from build123d import *

# Parameters (mm, degrees)
SKETCH1_R           = 3.2639
BOSS_EXTRUDE1_DEPTH = 6.35
FILLET2_R           = 6.35
FILLET3_R           = 2.54
FILLET6_R           = 6.35
FILLET7_R           = 6.35


with BuildPart() as part:
    # Sketch1 → Boss-Extrude1 (new, symmetric)
    with BuildSketch(Plane.XY):
        with BuildLine():
            ThreePointArc((1657.362226857, -25.665303386), (1645.082138382, -19.376819434), (1639.161234094, -31.838299916))
            Line((1639.161234094, -31.838299916), (1543.928298612, -110.961407638))
            Line((1543.928298612, -110.961407638), (1542.386268966, -109.105413681))
            Line((1542.386268966, -109.105413681), (1475.716388889, -164.497259751))
            ThreePointArc((1475.716388889, -164.497259751), (1463.735668917, -172.561408735), (1473.270132637, -183.40862734))
            Line((1473.270132637, -183.40862734), (1482.795132637, -183.40862734))
            Line((1482.795132637, -183.40862734), (1536.006430236, -216.269775409))
            Line((1536.006430236, -216.269775409), (1475.438186342, -259.678478553))
            ThreePointArc((1475.438186342, -259.678478553), (1465.455879345, -274.64513078), (1482.83634148, -270.00113812))
            Line((1482.83634148, -270.00113812), (1554.239311773, -218.827286252))
            Line((1554.239311773, -218.827286252), (1553.129588502, -217.278887316))
            Line((1553.129588502, -217.278887316), (1710.323691942, -104.61931964))
            Line((1710.323691942, -104.61931964), (1709.583876428, -103.587053683))
            Line((1709.583876428, -103.587053683), (1795.041714347, -42.340207499))
            ThreePointArc((1795.041714347, -42.340207499), (1809.776954687, -31.712536315), (1791.625246623, -30.944293485))
            Line((1791.625246623, -30.944293485), (1657.362226857, -25.665303386))
        make_face()
        with BuildLine():
            Line((1700.720652168, -102.126820321), (1556.109252329, -109.096723899))
            Line((1556.109252329, -109.096723899), (1643.219206848, -36.72249454))
            ThreePointArc((1643.219206848, -36.72249454), (1647.101886478, -38.035715693), (1651.178708707, -37.612311142))
            Line((1651.178708707, -37.612311142), (1700.720652168, -102.126820321))
        make_face(mode=Mode.SUBTRACT)
        with BuildLine():
            ThreePointArc((1482.659265028, -175.861431519), (1482.859244436, -174.484660756), (1482.858420935, -173.093442291))
            Line((1482.858420935, -173.093442291), (1541.633109373, -124.261218638))
            Line((1541.633109373, -124.261218638), (1541.60005002, -212.260879574))
            Line((1541.60005002, -212.260879574), (1482.659265028, -175.861431519))
        make_face(mode=Mode.SUBTRACT)
        with Locations((1473.270132637, -269.04472734)):
            Circle(SKETCH1_R, mode=Mode.SUBTRACT)
        with Locations((1473.270132637, -173.79472734)):
            Circle(SKETCH1_R, mode=Mode.SUBTRACT)
        Polygon((1547.986271365, -115.845602263), (1688.873329523, -109.05520253), (1547.950879905, -210.053025619), align=None, mode=Mode.SUBTRACT)
        with Locations((1648.169999473, -28.481334088)):
            Circle(SKETCH1_R, mode=Mode.SUBTRACT)
        with BuildLine():
            Line((1705.884798859, -98.425723899), (1656.215061092, -33.744798419))
            ThreePointArc((1656.215061092, -33.744798419), (1656.708059099, -32.900452896), (1657.112748585, -32.010400752))
            Line((1657.112748585, -32.010400752), (1791.19818023, -37.282408394))
            Line((1791.19818023, -37.282408394), (1705.884798859, -98.425723899))
        make_face(mode=Mode.SUBTRACT)
        with Locations((1800.567995736, -34.473360149)):
            Circle(SKETCH1_R, mode=Mode.SUBTRACT)
    extrude(amount=BOSS_EXTRUDE1_DEPTH, both=True)

    # Fillet2
    fillet2_edges = [part.edges().sort_by_distance(p)[0] for p in [
        (1541.60005002, -212.260879574, 0),
        (1547.986271365, -115.845602263, 0),
        (1700.720652168, -102.126820321, 0),
        (1791.625246623, -30.944293485, 0),
        (1795.041714347, -42.340207499, 0),
        (1482.83634148, -270.00113812, 0),
        (1475.438186342, -259.678478553, 0),
        (1475.716388889, -164.497259751, 0),
        (1639.161234094, -31.838299916, 0),
        (1657.362226857, -25.665303386, 0),
    ]]
    fillet(fillet2_edges, radius=FILLET2_R)

    # Fillet3
    # the kernel refuses this fillet: 2.54 mm, written as the material it adds along each edge
    with BuildSketch(Plane(origin=(1482.659265028, -175.861431519, -6.35), x_dir=(0.8508312617816599, -0.5254390202250196, 0), z_dir=(0, 0, 1)), Plane(origin=(1656.215061092, -33.744798419, -6.35), x_dir=(0.6090571217254737, -0.7931263597154502, 0), z_dir=(0, 0, 1))) as fillet3_piece_1:
        with BuildLine():
            CenterArc((1.651924419, 2.54), FILLET3_R, 208.048541525, 61.951458475)
            ThreePointArc((-0.5897514, 1.345642633), (-0.269132792, 0.684103596), (0, 0))
            Line((0, 0), (1.651924419, 0))
        make_face()
    extrude(amount=12.7)
    with BuildSketch(Plane(origin=(1541.633109373, -124.261218638, -6.35), x_dir=(-0.00037567588921249087, -0.9999999294338106, 0), z_dir=(0, 0, 1))) as fillet3_piece_2:
        with BuildLine():
            CenterArc((FILLET3_R * 2.13199085195, -FILLET3_R), FILLET3_R, 90, 129.742603087)
            Line((FILLET3_R * 1.36306647439, -FILLET3_R * 1.63933973879), (0, 0))
            Line((0, 0), (FILLET3_R * 2.13199085195, 0))
        make_face()
    extrude(amount=12.7)
    with BuildSketch(Plane(origin=(1547.950879905, -210.053025619, 6.35), x_dir=(0.8128078399508512, 0.5825319006839296, 0), z_dir=(0, 0, -1))) as fillet3_piece_3:
        with BuildLine():
            CenterArc((FILLET3_R * 1.94789411365, -FILLET3_R), FILLET3_R, 90, 125.650345443)
            Line((FILLET3_R * 1.13530517425, -FILLET3_R * 1.58283721188), (0, 0))
            Line((0, 0), (FILLET3_R * 1.94789411365, 0))
        make_face()
    extrude(amount=12.7)
    with BuildSketch(Plane(origin=(1688.873329523, -109.05520253, -6.35), x_dir=(-0.9988405216590461, -0.04814158588875568, 0), z_dir=(0, 0, 1))) as fillet3_piece_4:
        with BuildLine():
            CenterArc((FILLET3_R * 3.39012199782, FILLET3_R), FILLET3_R, 122.869444547, 147.130555453)
            Line((FILLET3_R * 2.8473953887, FILLET3_R * 1.83990941639), (0, 0))
            Line((0, 0), (FILLET3_R * 3.39012199782, 0))
        make_face()
    extrude(amount=12.7)
    with BuildSketch(Plane(origin=(1705.884798859, -98.425723899, -6.35), x_dir=(-0.6090571217254714, 0.7931263597154518, 0), z_dir=(0, 0, 1))) as fillet3_piece_5:
        with BuildLine():
            CenterArc((FILLET3_R * 0.967502749894, -FILLET3_R), FILLET3_R, 90, 88.10746289)
            Line((-FILLET3_R * 0.0319517760986, -FILLET3_R * 0.966975002291), (0, 0))
            Line((0, 0), (FILLET3_R * 0.967502749894, 0))
        make_face()
    extrude(amount=12.7)
    with BuildSketch(Plane(origin=(1791.19818023, -37.282408394, 6.35), x_dir=(-0.9992279317494432, 0.03928791686676534, 0), z_dir=(0, 0, -1))) as fillet3_piece_6:
        with BuildLine():
            CenterArc((FILLET3_R * 2.91408494962, -FILLET3_R), FILLET3_R, 90, 142.119567883)
            Line((FILLET3_R * 2.30006927648, -FILLET3_R * 1.78929383194), (0, 0))
            Line((0, 0), (FILLET3_R * 2.91408494962, 0))
        make_face()
    extrude(amount=12.7)
    with BuildSketch(Plane(origin=(1657.112748585, -32.010400752, -6.35), x_dir=(-0.4370826010652276, -0.8994213694626424, 0), z_dir=(0, 0, 1))) as fillet3_piece_7:
        with BuildLine():
            CenterArc((1.663286591, 2.532574185), FILLET3_R, 203.666275918, 61.951458475)
            Line((-0.663096919, 1.512995956), (0, 0))
            ThreePointArc((0, 0), (0.734602071, 0.02810671), (1.469204142, 0))
        make_face()
    extrude(amount=12.7)
    with BuildSketch(Plane(origin=(1556.109252329, -109.096723899, 6.35), x_dir=(0.9988405216590459, 0.048141585888763216, 0), z_dir=(0, 0, -1))) as fillet3_piece_8:
        with BuildLine():
            CenterArc((FILLET3_R * 2.99200774925, -FILLET3_R), FILLET3_R, 90, 143.038297809)
            Line((FILLET3_R * 2.39072668673, -FILLET3_R * 1.79903759853), (0, 0))
            Line((0, 0), (FILLET3_R * 2.99200774925, 0))
        make_face()
    extrude(amount=12.7)
    with BuildSketch(Plane(origin=(1651.178708707, -37.612311142, -6.35), x_dir=(0.6090571217254943, -0.7931263597154341, 0), z_dir=(0, 0, 1))) as fillet3_piece_9:
        with BuildLine():
            CenterArc((1.651924419, -2.54), FILLET3_R, 90, 61.951458475)
            ThreePointArc((-0.5897514, -1.345642633), (-0.269132792, -0.684103596), (0, 0))
            Line((0, 0), (1.651924419, 0))
        make_face()
    extrude(amount=12.7)
    with BuildSketch(Plane(origin=(1536.006430236, -216.269775409, -6.35), x_dir=(-0.8508312617816903, 0.5254390202249702, 0), z_dir=(0, 0, 1))) as fillet3_piece_10:
        with BuildLine():
            CenterArc((FILLET3_R * 1.50151874055, FILLET3_R), FILLET3_R, 157.326623381, 112.673376619)
            Line((FILLET3_R * 0.578801433411, FILLET3_R * 1.38547732891), (0, 0))
            Line((0, 0), (FILLET3_R * 1.50151874055, 0))
        make_face()
    extrude(amount=12.7)

    # Fillet6
    # the kernel refuses this fillet: 6.35 mm, written as the material it adds along each edge
    with BuildSketch(Plane(origin=(1543.928298612, -110.961407638, -6.35), x_dir=(-0.6390508273261215, 0.7691645078224811, 0), z_dir=(0, 0, 1))) as fillet6_piece_1:
        with BuildLine():
            CenterArc((6.35, -4.982221492), FILLET6_R, 128.316134474, 51.683865526)
            Line((0, -4.982221492), (-0.127, -4.982221492))
            Line((-0.127, -4.982221492), (-0.127, 0))
            Line((-0.127, 0), (0, 0.127))
            ThreePointArc((0, 0.127), (1.2065, 0.127), (2.33426, 0.09964443))
            Line((2.33426, 0.09964443), (2.413, 0))
        make_face()
    extrude(amount=12.7)
    with BuildSketch(Plane(origin=(1709.583876428, -103.587053683, 6.35), x_dir=(0.8128078399508694, 0.582531900683904, 0), z_dir=(0, 0, -1))) as fillet6_piece_2:
        with BuildLine():
            CenterArc((3.81, 6.35), FILLET6_R, 233.130102354, 36.869897646)
            Line((0, 1.27), (-0.0762, 1.1684))
            ThreePointArc((-0.0762, 1.1684), (-0.127, 0.635), (-0.127, 0))
            Line((-0.127, 0), (0, -0.127))
            Line((0, -0.127), (3.81, -0.127))
            Line((3.81, -0.127), (3.81, 0))
        make_face()
    extrude(amount=12.7)
    with BuildSketch(Plane(origin=(1553.129588502, -217.278887316, -6.35), x_dir=(0.8128078399508519, 0.5825319006839285, 0), z_dir=(0, 0, 1))) as fillet6_piece_3:
        with BuildLine():
            CenterArc((4.534807052, -6.35), FILLET6_R, 90, 45.572995999)
            Line((0, -1.905), (-0.090696141, -1.8161))
            ThreePointArc((-0.090696141, -1.8161), (-0.127, -0.9525), (-0.127, 0))
            Line((-0.127, 0), (0, 0.127))
            Line((0, 0.127), (4.534807052, 0.127))
            Line((4.534807052, 0.127), (4.534807052, 0))
        make_face()
    extrude(amount=12.7)

    # Fillet7
    fillet7_edges = [part.edges().sort_by_distance(p)[0] for p in [
        (1710.323691942, -104.61931964, 0),
        (1554.239311773, -218.827286252, 0),
        (1542.386268966, -109.105413681, 0),
    ]]
    fillet(fillet7_edges, radius=FILLET7_R)


solid = part.part
Can you work these out from the model? Positions are in its coordinate system, mm. A direction names the side the tool comes from. Round coordinates to 2 decimals unless told otherwise and drop trailing zeros. Order: outer loops, then holes, each group sorted by start corner. A loop starts at its lowest first (then second) coordinate and runs counter-clockwise, first axis right, second up. Notation, with made-up numbers: (-40, 57) - (-23, 57) arc R19 cw to (-23, 63) - close; hole circle Ø1 at (44, 83). An arc over 180 degrees is marked (long way). Answer in a Markdown table with one row per item.
(1) For P1, Ø5, axis at x = 1565, z = 1, coming from the +Y side; P2, Ø2, axis at y = -184.5, z = -1, coming from the -X side; P3, Ø6.5, axis at y = -160, z = 0, coming from the -X side, each with a flat end and sliding along its axis, tell me the tip position at first contact or that it passes through.
From the geometry:
| item | result |
|---|---|
| P1 | stops at y = -91.38 |
| P2 | stops at x = 1482.94 |
| P3 | stops at x = 1477.12 |
(2) Suppose I cut it at C-C, the plane z = -2.75. Count the separate pieces of the cut face and the enclosed holes in it, plus the area to 3 significant figures.
From the geometry:
| item | result |
|---|---|
| separate pieces | 1 |
| enclosed holes | 8 |
| area | 9,640 mm2 |
(3) Suppose I cut it at A-A, the plane x = 1668.5. Please give me the cut outline in (y, z), plus the area to 3 significant figures.
From the geometry:
| item | result |
|---|---|
| outline | (-134.59, -6.35) - (-123.66, -6.35) - (-123.66, 6.35) - (-134.59, 6.35) - close; (-110.04, -6.35) - (-103.68, -6.35) - (-103.68, 6.35) - (-110.04, 6.35) - close; (-60.17, -6.35) - (-49.74, -6.35) - (-49.74, 6.35) - (-60.17, 6.35) - close; (-32.46, -6.35) - (-26.1, -6.35) - (-26.1, 6.35) - (-32.46, 6.35) - close |
| area | 433 mm2 |
(4) If we mould it in two halves opening along Y, with no side actions, what happens to faces 1 (the face through (1518.186, -244.667, 0.089)), 2 (the face through (1725.38, -28.34, 0.09)), 3 (the face through (1617.83, -159.97, 0.09))? For each: released by +Y, released by -Y, zero draft, split by the parting line, or undercut.
From the geometry:
| item | result |
|---|---|
| face 1 | released by -Y |
| face 2 | released by +Y |
| face 3 | undercut |
(5) Which directions (+Z, -Z, +X, -X, +Y, -Y) give clear straight access to the entire face, cutting with the end or side of a thin tool? Please do faces 4 (the face through (1508.326, -191.712, 0.089)), 5 (the face through (1625, -107, 6.35)), 6 (the face through (1507.43, -198.62, 0.09)).
From the geometry:
| item | result |
|---|---|
| face 4 | +Z, -Z |
| face 5 | +Z, +X, -X, +Y, -Y |
| face 6 | +Z, -Z, -X |
(6) Suppose I cut it at B-B, the plane y = -71.5. Please give me the cut outline in (x, z) (3 decimals), plus the area to 3 significant figures.
From the geometry:
| item | result |
|---|---|
| outline | (1591.424, -6.35) - (1601.361, -6.35) - (1601.361, 6.35) - (1591.424, 6.35) - close; (1677.202, -6.35) - (1685.208, -6.35) - (1685.208, 6.35) - (1677.202, 6.35) - close; (1743.454, -6.35) - (1754.355, -6.35) - (1754.355, 6.35) - (1743.454, 6.35) - close |
| area | 366 mm2 |
(7) Please list where these lines run through material, in increasing order: L1, parallel to Y at x = 1518, z = -3.5; L2, parallel to Y at x = 1648.17, z = 3.75; L3, parallel to X at y = -142, z = -3.25. Write a range as from..to.
From the geometry:
| item | result |
|---|---|
| L1 | y = -244.8..-229.17, -205.15..-197.69, -143.9..-129.37 |
| L2 | y = -149.16..-138.23, -111.02..-104.66, -38.1..-31.75, -25.22..-18.87 |
| L3 | x = 1502.79..1520.28, 1541.63..1547.98, 1642.91..1658.17 |
